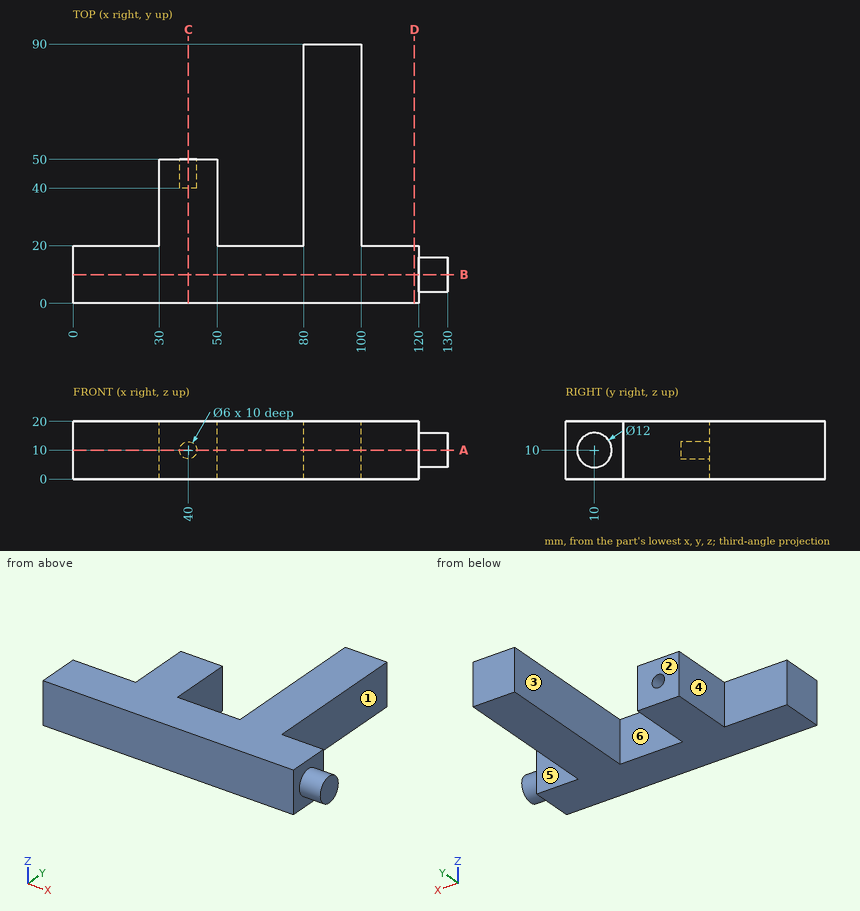
Check sheet for the drawn part. Datum: minimum x, y, z corner. Units: mm. A direction names the side the tool comes from. Round coordinates to 2 decimals unless told otherwise and drop trailing zeros. Loops run counter-clockwise (first coordinate to the right, second up) from the corner with the lowest first, then second, coordinate; pieces in that order, holes last. Notation, with made-up numbers: (79.25, 73) -> (85.25, 73) arc R22 cw to (85.25, 80) -> close; hole circle Ø4 at (56, 70). An arc over 180 degrees is marked (long way). Put each result on its own line as item: value. Start each with the question number.
1. Gauge pin test, flat ends, axial feed: pin 1 (1 mm diameter, centred on y = 76, z = 4, fed in from +X); pin 2 (10 mm diameter, centred on y = 71, z = 6.5, fed in from -X); pin 3 (6 mm diameter, centred on x = 71, z = 14, fed in from +Y). Record the tip position at first contact, or that the pin passes through.
2. Section check C-C (x = 40). Enter the section's corners in (y, z).
3. Section check B-B (y = 10). Enter the section's corners in (x, z).
4. Draft check along X on the marked faces 1, 2 and 3. Enter one of: +X half, -X half, draft (parallel to the pull), parting line (faces both ways), or undercut.
5. Section check D-D (x = 118.5). Enter the section's corners in (y, z), plus the area to 3 significant figures.
6. Section check A-A (z = 10). Enter the section's corners in (x, y).
7. Access from +Z, -Z, +X, -X, +Y, -Y to the whole of each face (thin tool, end or side, straight path). Record for the marked faces 4, 5 and 6.
8. Scan lines: probe 1 along X at (y, z) = (45.5, 10); probe 2 along X at (y, z) = (24.5, 6.75); probe 3 along Y at (x, z) = (8.5, 4.75). Record each from-to range of solid material in increasing order.
Findings:
1. pin 1: stops at x = 100
1. pin 2: stops at x = 80
1. pin 3: stops at y = 20
2. outline: (0, 0) -> (50, 0) -> (50, 7) -> (40, 7) -> (40, 13) -> (50, 13) -> (50, 20) -> (0, 20) -> close
3. outline: (0, 0) -> (120, 0) -> (120, 4) -> (130, 4) -> (130, 16) -> (120, 16) -> (120, 20) -> (0, 20) -> close
4. face 1: +X half
4. face 2: draft
4. face 3: undercut
5. outline: (0, 0) -> (20, 0) -> (20, 20) -> (0, 20) -> close
5. area: 400 mm^2
6. outline: (0, 0) -> (120, 0) -> (120, 4) -> (130, 4) -> (130, 16) -> (120, 16) -> (120, 20) -> (100, 20) -> (100, 90) -> (80, 90) -> (80, 20) -> (50, 20) -> (50, 50) -> (43, 50) -> (43, 40) -> (37, 40) -> (37, 50) -> (30, 50) -> (30, 20) -> (0, 20) -> close
7. face 4: +Z, -Z, -X, +Y
7. face 5: +Z, -Z, +X, +Y
7. face 6: +Z, -Z, +Y
8. probe 1: x = 30 to 37, 43 to 50, 80 to 100
8. probe 2: x = 30 to 50, 80 to 100
8. probe 3: y = 0 to 20
